CAD build for the part. Positions are in the model's coordinates, mm. Face numbers are marked on the shaded views. A direction names the side the tool comes from. Round coordinates to 2 decimals unless told otherwise and drop trailing zeros. Loops run counter-clockwise (first coordinate to the right, second up) from the corner with the lowest first, then second, coordinate; pieces in that order, holes last. Notation, with made-up numbers: (-23.75, -34.75) -> (23.25, -34.75) arc R34 cw to (23.25, -4.75) -> close; hole circle Ø4 at (43.5, -28.5). An arc over 180 degrees is marked (long way). Answer as CSV lines item,"result".
```python
from build123d import *

# Parameters (mm, degrees)
PAD_DEPTH       = 53
SKETCH001_R     = 1.65
POCKET_DEPTH    = 15
SKETCH002_R     = 1.65
POCKET001_DEPTH = 16
SKETCH003_R     = 4.5
POCKET002_DEPTH = 0.4
FILLET_R        = 3
POCKET003_DEPTH = 6


with BuildPart() as part:
    # Sketch → Pad (new body, symmetric)
    with BuildSketch(Plane.XZ):
        with BuildLine():
            ThreePointArc((-15.795942, 84.915204), (-20.82658, 87.235391), (-25.324265, 84.000982))
            Line((-25.324265, 84.000982), (-62.791985, 0))
            Line((57.208015, 0), (-62.791985, 0))
            Line((57.208015, 10.293343), (57.208015, 0))
            Line((57.208015, 10.293343), (55.487286, 12.750799))
            Line((41.561701, 3), (55.487286, 12.750799))
            Line((-15.795942, 84.915204), (41.561701, 3))
        make_face()
        with BuildLine():
            Line((-48.769346, 24.073542), (-22.584454, 82.77892))
            ThreePointArc((-18.253399, 83.194475), (-20.540052, 84.249105), (-22.584454, 82.77892))
            Line((-18.253399, 83.194475), (25.480661, 20.735764))
            ThreePointArc((27.289141, 15), (26.826311, 18.007058), (25.480661, 20.735764))
            Line((27.289141, 15), (27.289141, 3))
            Line((-49.636644, 3), (27.289141, 3))
            Line((-49.636644, 20), (-49.636644, 3))
            ThreePointArc((-48.769346, 24.073542), (-49.417416, 22.082423), (-49.636644, 20))
        make_face(mode=Mode.SUBTRACT)
    extrude(amount=PAD_DEPTH, both=True)

    # Sketch001 (on Face3 of Pad) → Pocket (cut, symmetric)
    with BuildSketch(Plane(origin=(29.297859, 0, 20.514582), x_dir=(-0.573576, 0, 0.819152), z_dir=(0.819152, 0, 0.573576))):
        with Locations((-23.881356, -47)):
            Circle(SKETCH001_R)
        with Locations((-23.881356, 47)):
            Circle(SKETCH001_R)
    extrude(amount=POCKET_DEPTH, both=True, mode=Mode.SUBTRACT)

    # Sketch002 (on Face6 of Pocket) → Pocket001 (cut)
    with BuildSketch(Plane(origin=(0, 0, 0), x_dir=(1, 0, 0), z_dir=(0, 0, -1))):
        with Locations((-52.5, 51.5)):
            Circle(SKETCH002_R)
        with Locations((30, 51.5)):
            Circle(SKETCH002_R)
        with Locations((30, -51.5)):
            Circle(SKETCH002_R)
        with Locations((-52.5, -51.5)):
            Circle(SKETCH002_R)
    extrude(amount=-POCKET001_DEPTH, mode=Mode.SUBTRACT)

    # Sketch003 → Pocket002 (cut)
    with BuildSketch(Plane(origin=(0, 0, 0), x_dir=(-1, 0, 0), z_dir=(0, 0, -1))):
        with Locations((-50, 46)):
            Circle(SKETCH003_R)
        with Locations((56, 46)):
            Circle(SKETCH003_R)
        with Locations((-50, -46)):
            Circle(SKETCH003_R)
        with Locations((56, -46)):
            Circle(SKETCH003_R)
    extrude(amount=-POCKET002_DEPTH, mode=Mode.SUBTRACT)

    # Fillet
    fillet_edges = [part.edges().sort_by_distance(p)[0] for p in [
        (27.289141, 0, 3),
        (-49.636644, 0, 3),
    ]]
    fillet(fillet_edges, radius=FILLET_R)

    # Sketch004 (on Face5 of Fillet) → Pocket003 (cut, symmetric)
    with BuildSketch(Plane(origin=(0, 0, 3), x_dir=(-1, 0, 0), z_dir=(0, 0, 1))):
        with BuildLine():
            Line((-24.289141, 46.5), (46.636644, 46.5))
            ThreePointArc((49.636644, 43.5), (48.757964, 45.62132), (46.636644, 46.5))
            Line((49.636644, 43.5), (49.636644, -43.5))
            ThreePointArc((46.636644, -46.5), (48.757964, -45.62132), (49.636644, -43.5))
            Line((46.636644, -46.5), (-24.289141, -46.5))
            ThreePointArc((-27.289141, -43.5), (-26.410461, -45.62132), (-24.289141, -46.5))
            Line((-27.289141, -43.5), (-27.289141, 43.5))
            ThreePointArc((-24.289141, 46.5), (-26.410461, 45.62132), (-27.289141, 43.5))
        make_face()
    extrude(amount=POCKET003_DEPTH, both=True, mode=Mode.SUBTRACT)


solid = part.part
```
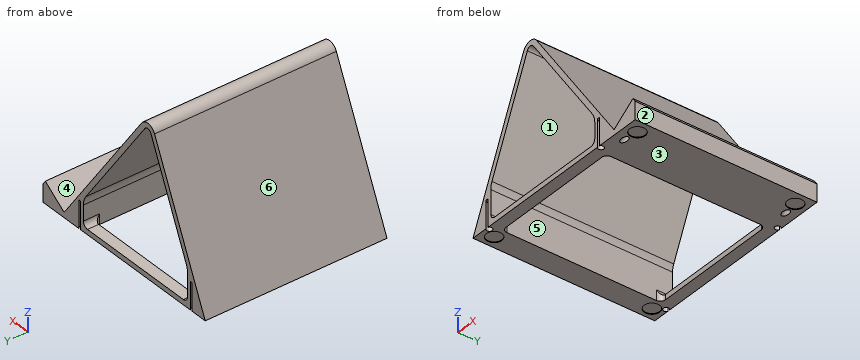
Q1. Drop flat-ended pins along their axis: pin 1 Ø4 at (y, z) = (-21, 19.5) entering from -X; pin 2 Ø2 at (x, y) = (1, 50.5) entering from +Z; pin 3 Ø2.5 at (x, y) = (-54.5, -45) entering from -Z; pin 4 Ø1.6 at (x, y) = (31, -51) entering from -Z. Give the stop position or say it passes through.
Results:
pin 1,"x = -54.99"
pin 2,"z = 62.36"
pin 3,"z = 0.4"
pin 4,"z = 0"
Q2. Tool access for the marked faces 4, 5 and 6: list every direction of +Z, -Z, +X, -X, +Y, -Y with a clear straight run to the whole face (end or side of a thin tool).
Results:
face 4,"+Z, +Y, -Y"
face 5,"none"
face 6,"+Z, -X, +Y, -Y"
Q3. Slice it at C-C, the plane y = -17. Give the cut face in (x, z).
Results:
outline,"(-62.79, 0) -> (-49.64, 0) -> (-49.64, 20) arc R10 cw to (-48.77, 24.07) -> (-22.58, 82.78) arc R2.5 cw to (-18.25, 83.19) -> (25.48, 20.74) arc R10 cw to (27.29, 15) -> (27.29, 0) -> (57.21, 0) -> (57.21, 10.29) -> (55.49, 12.75) -> (41.56, 3) -> (-15.8, 84.92) arc R5.5 ccw to (-25.32, 84) -> close"
Q4. Slice it at A-A, the plane z = 56.5. Give the cut face in (x, y).
Results:
outline,"(-37.59, -53) -> (-34.31, -53) -> (-34.31, 53) -> (-37.59, 53) -> close; (0.44, -53) -> (4.1, -53) -> (4.1, 53) -> (0.44, 53) -> close"
Q5. Slice it at D-D, the plane x = -40.5. Give the cut face in (y, z), and give its area (3 significant figures).
Results:
outline,"(-53, 0) -> (-46.5, 0) -> (-46.5, 3) -> (-53, 3) -> close; (-53, 42.61) -> (53, 42.61) -> (53, 49.98) -> (-53, 49.98) -> close; (46.5, 0) -> (53, 0) -> (53, 3) -> (46.5, 3) -> close"
area,"820 mm2"
Q6. Two-plate mould, pull along X, no slides. Class the marked faces 1, 2 and 3: pulls with the +X half, pulls with the -X half, needs draft (parallel to the pull), parting line crosses it, or undercut.
Results:
face 1,"undercut"
face 2,"pulls with the +X half"
face 3,"needs draft"
Q7. Probe L1, parallel to Y at x = 50, z = 0.1; L2, parallel to X at y = 25.5, z = 10; L3, parallel to X at y = -51.5, z = 9.5. List the from-to ranges inside material, lowest first. Write a range as [from, to].
Results:
L1,"[-53, -50.5], [-41.5, 41.5], [50.5, 53]"
L2,"[-58.33, -49.64], [27.29, 36.66], [51.56, 57.21]"
L3,"[-58.55, -54.15], [-50.85, -49.64], [27.29, 28.35], [31.65, 37.01], [50.84, 57.21]"
Q8. Slice it at B-B, the plane x = 8. Give the cut face in (y, z).
Results:
outline,"(-53, 0) -> (-46.5, 0) -> (-46.5, 3) -> (-53, 3) -> close; (-53, 45.7) -> (53, 45.7) -> (53, 50.93) -> (-53, 50.93) -> close; (46.5, 0) -> (53, 0) -> (53, 3) -> (46.5, 3) -> close"
